Could you check a few things on this model? Use its own coordinates, in mm. Round coordinates to 2 decimals unless told otherwise and drop trailing zeros. Loops run counter-clockwise (first coordinate to the right, second up) from the corner with the lowest first, then second, coordinate; pieces in that order, holes last.
from build123d import *

# Parameters (mm, degrees)
F0_W     = 200
F0_H     = 150
F0_R     = 3
F0_R_2   = 8.5
F1_DEPTH = 1.5


with BuildPart() as f1:
    # F0 (on Front) → F1 (new body, symmetric)
    with BuildSketch(Plane.XZ):
        Rectangle(F0_W, F0_H)
        with Locations((70, -50)):
            Circle(F0_R, mode=Mode.SUBTRACT)
        with Locations((70, 0)):
            Circle(F0_R_2, mode=Mode.SUBTRACT)
        with Locations((70, 50)):
            Circle(F0_R, mode=Mode.SUBTRACT)
    extrude(amount=F1_DEPTH, both=True)


solid = f1.part
Item 1: We'd pull the mould along Z, two halves only. Please class faces 1 (the flat face through (-1, -1.5, 1)), 2 (the cylindrical face through (67.79, 0.02, -47.97)): released by +Z, released by -Z, zero draft, split by the parting line, or undercut.
Results list:
face 1: zero draft
face 2: undercut
Item 2: Will this pin go through, and if not, where does the flat tip stop? pin 1 (3.5 mm diameter, centred on x = 70, z = 50, fed in from -Y).
Results list:
pin 1: passes through
Item 3: If we section it at B-B, the plane z = 50: Please give me the cut outline in (x, y), then the cut area to 3 significant figures.
Results list:
outline: (-100, -1.5) - (67, -1.5) - (67, 1.5) - (-100, 1.5) - close; (73, -1.5) - (100, -1.5) - (100, 1.5) - (73, 1.5) - close
area: 582 mm2
Item 4: If we section it at A-A, the plane x = 70: Please give me the cut outline in (y, z), then the cut area to 3 significant figures.
Results list:
outline: (-1.5, -75) - (1.5, -75) - (1.5, -53) - (-1.5, -53) - close; (-1.5, -47) - (1.5, -47) - (1.5, -8.5) - (-1.5, -8.5) - close; (-1.5, 8.5) - (1.5, 8.5) - (1.5, 47) - (-1.5, 47) - close; (-1.5, 53) - (1.5, 53) - (1.5, 75) - (-1.5, 75) - close
area: 363 mm2
Item 5: If I drill on line 1 along Z through (x, y) = (70, -0.65); line 2 along Z through (x, y) = (65, 0.6), over which ranges is the centre line in solid material (lowest first)?
Results list:
line 1: z = -75 to -53, -47 to -8.5, 8.5 to 47, 53 to 75
line 2: z = -75 to -6.87, 6.87 to 75
Item 6: If we section it at C-C, the plane z = 0: Please give me the cut outline in (x, y).
Results list:
outline: (-100, -1.5) - (61.5, -1.5) - (61.5, 1.5) - (-100, 1.5) - close; (78.5, -1.5) - (100, -1.5) - (100, 1.5) - (78.5, 1.5) - close
